from build123d import *

# Parameters (mm, degrees)
BOSS_EXTRUDE1_DEPTH = 1.5
BOSS_EXTRUDE2_DEPTH = 2.5
SKETCH3_R           = 2.625
BOSS_EXTRUDE3_DEPTH = 0.01
SKETCH4_W           = 3
SKETCH4_H           = 0.2
BOSS_EXTRUDE4_DEPTH = 1
SKETCH5_W           = 0.9
SKETCH5_H           = 0.2
BOSS_EXTRUDE5_DEPTH = 0.25
BOSS_EXTRUDE6_REACH = 17.786
SKETCH6_W           = 0.9
SKETCH6_H           = 0.2
SKETCH8_W           = 1.5
SKETCH8_H           = 4
BOSS_EXTRUDE7_DEPTH = 0.5
CIRPATTERN1_COUNT   = 2
CUT_EXTRUDE1_DEPTH  = 17.115258556
CIRPATTERN2_COUNT   = 6
CUT_EXTRUDE2_DEPTH  = 0.1


# Read off the part's stored shape, not the designer's step: Dome1
with BuildPart() as part:
    # Sketch1 → Boss-Extrude1 (new body)
    with BuildSketch(Plane(origin=(0, 0, 0), x_dir=(1, 0, 0), z_dir=(0, 1, 0))):
        Polygon((-11.547005384, 0), (-5.773502692, -10), (5.773502692, -10), (11.547005384, 0), (5.773502692, 10), (-5.773502692, 10), align=None)
    extrude(amount=BOSS_EXTRUDE1_DEPTH)

    # Sketch2 → Boss-Extrude2 (add)
    with BuildSketch(Plane(origin=(0, 1.5, 0), x_dir=(1, 0, 0), z_dir=(0, 1, 0))):
        with BuildLine():
            Line((-1.936491673, 3.5), (1.936491673, 3.5))
            ThreePointArc((1.936491673, 3.5), (4, 0), (1.936491673, -3.5))
            Line((1.936491673, -3.5), (-1.936491673, -3.5))
            ThreePointArc((-1.936491673, -3.5), (-4, 0), (-1.936491673, 3.5))
        make_face()
    extrude(amount=BOSS_EXTRUDE2_DEPTH)

    # Sketch3 → Boss-Extrude3 (add)
    with BuildSketch(Plane(origin=(0, 4, 0), x_dir=(1, 0, 0), z_dir=(0, 1, 0))):
        with Locations(Location((0, 0, 0), (0, 0, 90))):
            Circle(SKETCH3_R)
    extrude(amount=BOSS_EXTRUDE3_DEPTH)

    # Dome1 outline → Dome1 (revolve)
    with BuildSketch(Plane.XY):
        with BuildLine():
            Line((0, 4.01), (2.625, 4.009999997))
            ThreePointArc((2.625, 4.009999997), (1.856155302, 5.8661553), (0, 6.635))
            Line((0, 6.635), (0, 4.01))
        make_face()
    revolve(axis=Axis((0, 0, 0), (0, 1, 0)))

    # Sketch4 → Boss-Extrude4 (add)
    with BuildSketch(Plane.XY.offset(3.5)):
        with Locations((0, 2.75)):
            Rectangle(SKETCH4_W, SKETCH4_H)
    boss_extrude4 = extrude(amount=BOSS_EXTRUDE4_DEPTH)

    # Sketch5 → Boss-Extrude5 (add)
    with BuildSketch(Plane.XY.offset(4.5)):
        with Locations((1.05, 2.75)):
            Rectangle(SKETCH5_W, SKETCH5_H)
    boss_extrude5 = extrude(amount=BOSS_EXTRUDE5_DEPTH)

    # Sketch6 → Boss-Extrude6 (add, up to next)
    with BuildSketch(Plane.XZ.offset(-2.65), mode=Mode.PRIVATE) as boss_extrude6_sk1:
        with Locations((1.05, 4.65)):
            Rectangle(SKETCH6_W, SKETCH6_H)
    boss_extrude6_tool1 = extrude(boss_extrude6_sk1.sketch, amount=BOSS_EXTRUDE6_REACH, mode=Mode.PRIVATE) - part.part
    boss_extrude6 = boss_extrude6_tool1.solids().sort_by_distance((1.05, 2.65, 4.65))[0]
    add(boss_extrude6)

    # Sketch8 → Boss-Extrude7 (add)
    with BuildSketch(Plane(origin=(0, 1.5, 0), x_dir=(1, 0, 0), z_dir=(0, 1, 0))):
        with Locations((1.05, -6.5)):
            Rectangle(SKETCH8_W, SKETCH8_H)
    boss_extrude7 = extrude(amount=BOSS_EXTRUDE7_DEPTH)

    # CirPattern1: Boss-Extrude4, Boss-Extrude5, Boss-Extrude6, Boss-Extrude7 ×2 about axis
    cirpattern1_axis = Axis((0, 0, 0), (0, 1, 0))
    add([boss_extrude4.rotate(cirpattern1_axis, i * 360 / CIRPATTERN1_COUNT) for i in range(1, CIRPATTERN1_COUNT)])
    add([boss_extrude5.rotate(cirpattern1_axis, i * 360 / CIRPATTERN1_COUNT) for i in range(1, CIRPATTERN1_COUNT)])
    add([boss_extrude6.rotate(cirpattern1_axis, i * 360 / CIRPATTERN1_COUNT) for i in range(1, CIRPATTERN1_COUNT)])
    add([boss_extrude7.rotate(cirpattern1_axis, i * 360 / CIRPATTERN1_COUNT) for i in range(1, CIRPATTERN1_COUNT)])

    # Sketch9 → Cut-Extrude1 (cut, through all)
    with BuildSketch(Plane(origin=(0, 1.5, 0), x_dir=(1, 0, 0), z_dir=(0, 1, 0))):
        with BuildLine():
            Line((-6.200961894, 13.740381057), (-3.700961894, 9.410254038))
            ThreePointArc((-3.700961894, 9.410254038), (-4.25, 7.361215932), (-6.299038106, 7.910254038))
            Line((-6.299038106, 7.910254038), (-8.799038106, 12.240381057))
            ThreePointArc((-8.799038106, 12.240381057), (-8.25, 14.289419162), (-6.200961894, 13.740381057))
        make_face()
    cut_extrude1 = extrude(amount=-CUT_EXTRUDE1_DEPTH, mode=Mode.SUBTRACT)

    # CirPattern2: Cut-Extrude1 ×6 about axis
    cirpattern2_axis = Axis((0, 0, 0), (0, 1, 0))
    for i in range(1, CIRPATTERN2_COUNT):
        add(cut_extrude1.rotate(cirpattern2_axis, i * 360 / CIRPATTERN2_COUNT), mode=Mode.SUBTRACT)

    # Sketch10 → Cut-Extrude2 (cut)
    # profile 1 of 5: a face of its own
    with BuildSketch(Plane(origin=(0, 1.5, 0), x_dir=(1, 0, 0), z_dir=(0, 1, 0))):
        with BuildLine():
            Line((-6.639528096, 8.5), (-10.68097998, 1.5))
            Line((-10.68097998, 1.5), (-10, 1.5))
            ThreePointArc((-10, 1.5), (-8.5, 0), (-10, -1.5))
            Line((-10, -1.5), (-10.68097998, -1.5))
            Line((-10.68097998, -1.5), (-6.639528096, -8.5))
            Line((-6.639528096, -8.5), (-6.299038106, -7.910254038))
            ThreePointArc((-6.299038106, -7.910254038), (-4.25, -7.361215932), (-3.700961894, -9.410254038))
            Line((-3.700961894, -9.410254038), (-4.041451884, -10))
            Line((-4.041451884, -10), (4.041451884, -10))
            Line((4.041451884, -10), (3.700961894, -9.410254038))
            ThreePointArc((3.700961894, -9.410254038), (4.25, -7.361215932), (6.299038106, -7.910254038))
            Line((6.299038106, -7.910254038), (6.639528096, -8.5))
            Line((6.639528096, -8.5), (10.68097998, -1.5))
            Line((10.68097998, -1.5), (10, -1.5))
            ThreePointArc((10, -1.5), (8.5, 0), (10, 1.5))
            Line((10, 1.5), (10.68097998, 1.5))
            Line((10.68097998, 1.5), (6.639528096, 8.5))
            Line((6.639528096, 8.5), (6.299038106, 7.910254038))
            ThreePointArc((6.299038106, 7.910254038), (4.25, 7.361215932), (3.700961894, 9.410254038))
            Line((3.700961894, 9.410254038), (4.041451884, 10))
            Line((4.041451884, 10), (-4.041451884, 10))
            Line((-4.041451884, 10), (-3.700961894, 9.410254038))
            ThreePointArc((-3.700961894, 9.410254038), (-4.25, 7.361215932), (-6.299038106, 7.910254038))
            Line((-6.299038106, 7.910254038), (-6.639528096, 8.5))
        make_face()
        with BuildLine():
            ThreePointArc((-2.523193047, 9), (-3.75, 6.495190528), (-6.53263211, 6.685149278))
            Line((-6.53263211, 6.685149278), (-9.055825158, 2.314850722))
            ThreePointArc((-9.055825158, 2.314850722), (-7.5, 0), (-9.055825158, -2.314850722))
            Line((-9.055825158, -2.314850722), (-6.53263211, -6.685149278))
            ThreePointArc((-6.53263211, -6.685149278), (-3.75, -6.495190528), (-2.523193047, -9))
            Line((-2.523193047, -9), (2.523193047, -9))
            ThreePointArc((2.523193047, -9), (3.75, -6.495190528), (6.53263211, -6.685149278))
            Line((6.53263211, -6.685149278), (9.055825158, -2.314850722))
            ThreePointArc((9.055825158, -2.314850722), (7.5, 0), (9.055825158, 2.314850722))
            Line((9.055825158, 2.314850722), (6.53263211, 6.685149278))
            ThreePointArc((6.53263211, 6.685149278), (3.75, 6.495190528), (2.523193047, 9))
            Line((2.523193047, 9), (-2.523193047, 9))
        make_face(mode=Mode.SUBTRACT)
    # profile 2 of 5: a face of its own
    with BuildSketch(Plane(origin=(0, 1.5, 0), x_dir=(1, 0, 0), z_dir=(0, 1, 0))):
        Polygon((-7.835723618, 2.503231198), (-6.320179161, 1.628231198), (-4.570179161, 4.659320111), (-6.085723618, 5.534320111), align=None)
    # profile 3 of 5: a face of its own
    with BuildSketch(Plane(origin=(0, 1.5, 0), x_dir=(1, 0, 0), z_dir=(0, 1, 0))):
        Polygon((-6.320179161, -1.628231198), (-4.570179161, -4.659320111), (-6.085723618, -5.534320111), (-7.835723618, -2.503231198), align=None)
    # profile 4 of 5: a face of its own
    with BuildSketch(Plane(origin=(0, 1.5, 0), x_dir=(1, 0, 0), z_dir=(0, 1, 0))):
        Polygon((7.835723618, -2.503231198), (6.085723618, -5.534320111), (4.570179161, -4.659320111), (6.320179161, -1.628231198), align=None)
    # profile 5 of 5: a face of its own
    with BuildSketch(Plane(origin=(0, 1.5, 0), x_dir=(1, 0, 0), z_dir=(0, 1, 0))):
        Polygon((7.835723618, 2.503231198), (6.320179161, 1.628231198), (4.570179161, 4.659320111), (6.085723618, 5.534320111), align=None)
    extrude(amount=-CUT_EXTRUDE2_DEPTH, mode=Mode.SUBTRACT)


solid = part.part
Work out the finished part from the listing and answer in its coordinate system (mm). A direction names the side the tool comes from. Coordinates: 2 decimals unless noted, no trailing zeros. Write each loop counter-clockwise with the first axis right and the second up, starting at its lowest first coordinate (ties: lowest second). Pieces come first, ordered by that corner, then holes. Notation, with made-up numbers: (58, -34.75) - (109, -34.75) arc R24 cw to (109, -0.75) - close; hole circle Ø2 at (64.25, -25). An arc over 180 degrees is marked (long way). One line per question, with ' | ' between items.
1) Find section C-C, the plane z = 0. Determine the outline of the cut face in (x, y) (3 decimals).
Checks:
outline: (-8.5, 0) - (8.5, 0) - (8.5, 1.4) - (7.5, 1.4) - (7.5, 1.5) - (4, 1.5) - (4, 4) - (2.625, 4) - (2.625, 4.01) arc R2.625 ccw to (-2.625, 4.01) - (-2.625, 4) - (-4, 4) - (-4, 1.5) - (-7.5, 1.5) - (-7.5, 1.4) - (-8.5, 1.4) - close
2) Find section B-B, the plane x = 0. Determine the outline of the cut face in (y, z) (3 decimals), and give its area (3 significant figures).
Checks:
outline: (0, -10) - (1.4, -10) - (1.4, -9) - (1.5, -9) - (1.5, -3.5) - (2.65, -3.5) - (2.65, -4.5) - (2.85, -4.5) - (2.85, -3.5) - (4, -3.5) - (4, -2.625) - (4.01, -2.625) arc R2.625 ccw to (4.01, 2.625) - (4, 2.625) - (4, 3.5) - (2.85, 3.5) - (2.85, 4.5) - (2.65, 4.5) - (2.65, 3.5) - (1.5, 3.5) - (1.5, 9) - (1.4, 9) - (1.4, 10) - (0, 10) - close | area: 58.6 mm2
3) Flat-ended cylindrical pins translate along their axes: P1, Ø1.5, axis at x = 0.5, y = 2.5, coming from the +Z side; P2, Ø0.6, axis at x = -1, y = 2, coming from the +Z side; P3, Ø0.8, axis at x = -1, y = 3, coming from the +Z side. Find the tip coordinate at first contact, or state that the pin passes through.
Checks:
P1: z = 8.5 | P2: z = 3.5 | P3: z = 4.5
4) Find section D-D, the plane y = 5. Determine the outline of the cut face in (x, z), and give its area (3 significant figures).
Checks:
outline: circle Ø4.86 at (0, 0) | area: 18.6 mm2
5) Find section A-A, the plane y = 1.75. Determine the outline of the cut face in (x, z).
Checks:
outline: (-1.94, -3.5) - (1.94, -3.5) arc R4 ccw to (1.94, 3.5) - (-1.94, 3.5) arc R4 ccw to start; (-1.8, -8.5) - (-0.3, -8.5) - (-0.3, -4.5) - (-1.8, -4.5) - close; (0.3, 4.5) - (1.8, 4.5) - (1.8, 8.5) - (0.3, 8.5) - close
6) For faces 4 (the face through (-6, 1.4, 4)), 5 (the face through (0, 2.65, -4)), determine the directions among +Z, -Z, +X, -X, +Y, -Y from which every point of the face is accessible in a straight line to the end or side of a thin tool.
Checks:
face 4: +Y | face 5: +X, -X
7) The mould has two halves that part along X. Classify faces 1 (the face through (3, 4, 0)), 2 (the face through (-4.22, 0.71, -7.38)), 3 (the face through (-8.63, 0.69, -5.05)): +X half, -X half, draft (parallel to the pull), parting line (faces both ways), or undercut.
Checks:
face 1: draft | face 2: undercut | face 3: -X half
8) Consider probe 1 along Z at (x, y) = (-0.5, 1.75); probe 2 along Y at (x, z) = (-6.5, 7.5); probe 3 along Y at (x, z) = (-6.75, 5.5). Determine where each line is inside the solid, lowest interval first. Write a range as [from, to].
Checks:
probe 1: [-8.5, -4.5], [-3.5, 3.5] | probe 2: [0, 1.4] | probe 3: [0, 1.5]
